Can you work these out from the model? Positions are in its coordinate system, mm. Coordinates: 2 decimals unless noted, no trailing zeros. Order: outer loops, then holes, each group sorted by start corner. A loop starts at its lowest first (then second) coordinate and runs counter-clockwise, first axis right, second up. Notation, with made-up numbers: (-27, -8.75) - (-16, -8.75) arc R21 cw to (-16, 17.25) - close; hole circle Ø6 at (-6, 48). An arc over 180 degrees is marked (long way). Use a Markdown table: item, result. Add a question column.
(1) If I drill on L1, parallel to Z at x = 3.75, y = 2.75; L2, parallel to Y at x = 6.75, z = 3.75; L3, parallel to X at y = 5.5, z = 6.75, over which ranges is the centre line in solid material (lowest first)? Write a range as [from, to].
(2) For pin 1 Ø5 at (y, z) = (8.5, 3) entering from -X; pin 2 Ø3 at (x, z) = (10.5, 2.5) entering from -Y, each with a flat end and sliding along its axis, tell me the tip position at first contact or that it passes through.
(3) I want a section at A-A (z = 5.5). List the corners of the cut face in (x, y) for me (3 decimals), and give its area (3 significant figures).
(4) I want a section at B-B (x = 7.25). List the corners of the cut face in (y, z) for me.
(5) I want a section at C-C (y = 4.75). List the corners of the cut face in (x, z) for me.
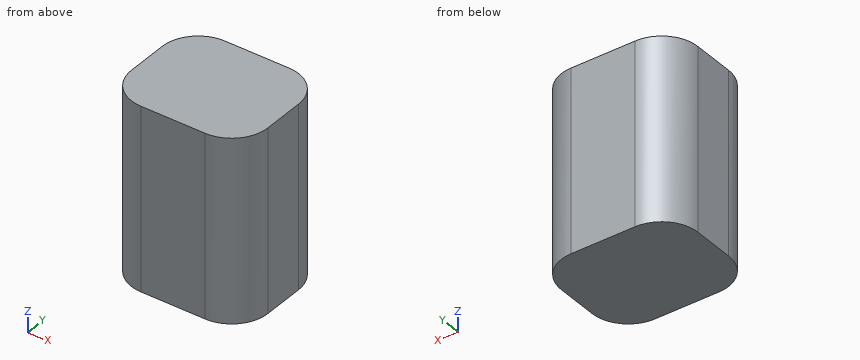
Autodesk Inventor part; units mm, degrees
ref_plane "YZ Plane" through (0, 0, 0) normal (1, 0, 0) x (0, 1, 0)
ref_plane "XZ Plane" through (0, 0, 0) normal (0, 1, 0) x (-1, 0, 0)
ref_plane "XY Plane" through (0, 0, 0) normal (0, 0, 1) x (1, 0, 0)
sketch "Sketch1" plane through (0, 0, 0) normal (0, 0, 1) x (1, 0, 0)
  line L0 (0, 0) -> (11.9888, 0)
  line L1 (11.9888, 0) -> (11.9888, 10.0076)
  line L2 (11.9888, 10.0076) -> (0, 10.0076)
  line L3 (0, 10.0076) -> (0, 0)
  dimension "d0" = 10.0076
  dimension "d1" = 11.9888
extrude "Extrusion1" add sketch "Sketch1" along normal blind 16.002
fillet "Fillet1" radius 3.175 4 edges at (11.9888, 10.0076, 8.001) (0, 10.0076, 8.001) (11.9888, 0, 8.001) (0, 0, 8.001)
shell "Shell2" thickness 0.254 removed faces 0
properties part number "Gearmotor_Motor" material "Stainless Steel"
Answers follow:
| question | item | result |
|---|---|---|
| 1 | L1 | z = [0, 0.25], [15.75, 16] |
| 1 | L2 | y = [0, 0.25], [9.75, 10.01] |
| 1 | L3 | x = [0, 0.25], [11.73, 11.99] |
| 2 | pin 1 | stops at x = 0 |
| 2 | pin 2 | stops at y = 0.01 |
| 3 | outline | (0, 3.175) arc R3.175 ccw to (3.175, 0) - (8.814, 0) arc R3.175 ccw to (11.989, 3.175) - (11.989, 6.833) arc R3.175 ccw to (8.814, 10.008) - (3.175, 10.008) arc R3.175 ccw to (0, 6.833) - close; hole (0.254, 3.175) arc R2.921 ccw to (3.175, 0.254) - (8.814, 0.254) arc R2.921 ccw to (11.735, 3.175) - (11.735, 6.833) arc R2.921 ccw to (8.814, 9.754) - (3.175, 9.754) arc R2.921 ccw to (0.254, 6.833) - close |
| 3 | area | 9.59 mm² |
| 4 | outline | (0, 0) - (10.01, 0) - (10.01, 16) - (0, 16) - close; hole (0.25, 0.25) - (9.75, 0.25) - (9.75, 15.75) - (0.25, 15.75) - close |
| 5 | outline | (0, 0) - (11.99, 0) - (11.99, 16) - (0, 16) - close; hole (0.25, 0.25) - (11.73, 0.25) - (11.73, 15.75) - (0.25, 15.75) - close |
